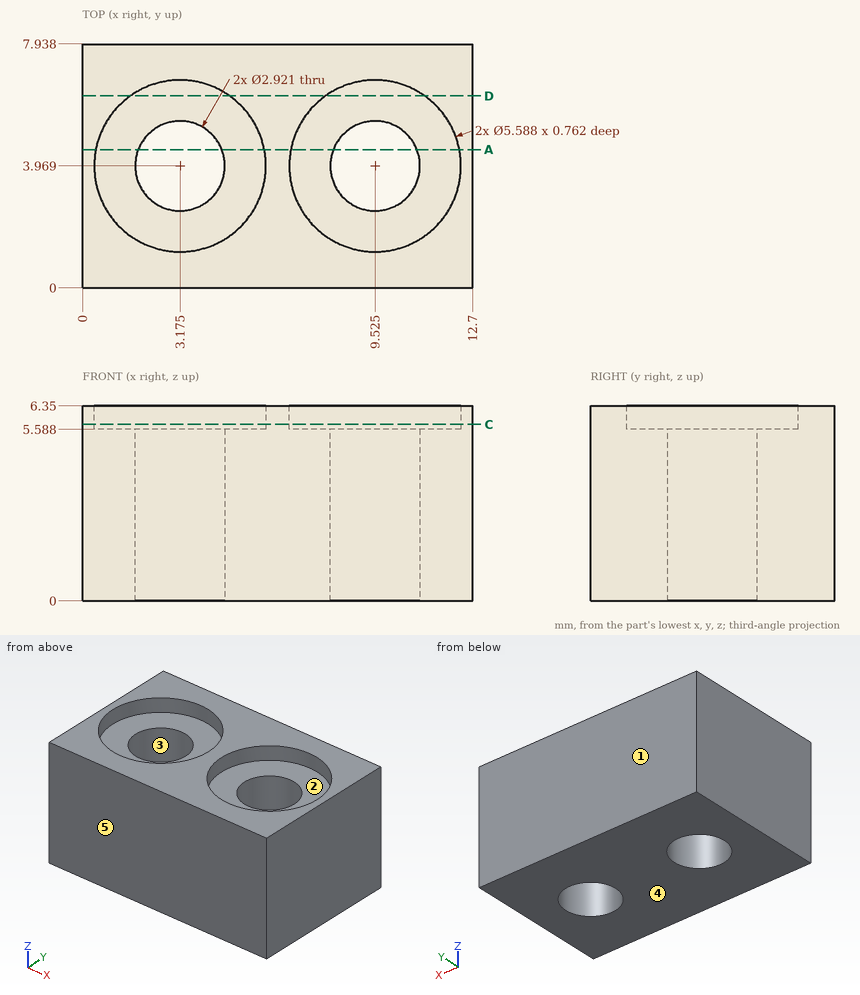
Job drawing, mm, ordinate dimensions from the low corner. One solid piece. A direction names the side the tool comes from. Give positions to 0.01 mm unless a question says otherwise; leave off trailing zeros. Loops run counter-clockwise (first coordinate to the right, second up) from the corner with the lowest first, then second, coordinate; pieces in that order, holes last. Notation, with made-up numbers: M 69.25,62 L 99.25,62 A12 ccw 99.25,77 Z; hole C 48.25,48.25 d11. An arc over 180 degrees is marked long. Use one line per item in the form item = value.
Item 1: Slice it at A-A on y = 4.5. Give the number of separate pieces and of enclosed holes in the cut face.
Filled in:
separate_pieces = 3
enclosed_holes = 0
Item 2: Slice it at D-D on y = 6.25. List the corners of the cut face in (x, z).
Filled in:
outline = M 0,0 L 12.7,0 L 12.7,6.35 L 11.14,6.35 L 11.14,5.59 L 7.91,5.59 L 7.91,6.35 L 4.79,6.35 L 4.79,5.59 L 1.56,5.59 L 1.56,6.35 L 0,6.35 Z
Item 3: Flat gauge pins, fed straight in: pin 1 Ø2.5 at (x, y) = (9.52, 3.97) entering from +Z; pin 2 Ø1.5 at (x, y) = (8.5, 3.5) entering from +Z. Where does each tip first touch, or does it go through?
Filled in:
pin_1 = through
pin_2 = 5.59
Item 4: Slice it at C-C on z = 5.75. List the corners of the cut face in (x, y) (1 decimal).
Filled in:
outline = M 0,0 L 12.7,0 L 12.7,7.9 L 0,7.9 Z; hole C 3.2,4 d5.6; hole C 9.5,4 d5.6
Item 5: Drill centre lines: L1, parallel to X at y = 4, z = 2.5 (1 decimal); L2, parallel to Y at x = 3.25, z = 3.75; L3, parallel to X at y = 2.5, z = 6. Where is each one in solid material? Low to high.
Filled in:
L1 = 0 to 1.7, 4.6 to 8.1, 11 to 12.7
L2 = 0 to 2.51, 5.43 to 7.94
L3 = 0 to 0.8, 5.55 to 7.15, 11.9 to 12.7
Item 6: Two-plate mould, pull along Y, no slides. Class the marked faces 3, 4 and 5: released by +Y, released by -Y, zero draft, split by the parting line, or undercut.
Filled in:
face_3 = undercut
face_4 = zero draft
face_5 = released by -Y
Item 7: Which spindle directions (+Z, -Z, +X, -X, +Y, -Y) get a long thin tool onto all of the face, cutting with end or side? Do the marked faces 1 and 2. Say none if no direction does.
Filled in:
face_1 = +Z, -Z, +X, -X, +Y
face_2 = +Z
